```python
from build123d import *

# Parameters (mm, degrees)
FILLET1_R     = 1
CHAMFER1_SIZE = 0.5


with BuildPart() as part:
    # Sketch1 → Revolve1 (revolve)
    with BuildSketch(Plane.XY, mode=Mode.PRIVATE) as revolve1_sk:
        Polygon((-26, 0), (-22.5, 0), (-22.5, 2.872417267), (-15.5, 11.5), (-13, 11.5), (-13, 19.5), (-15.142082361, 19.5), (-25, 7.35), (-25, 1), (-26, 1), align=None)
    revolve(revolve1_sk.sketch.rotate(Axis((0, 0, 0), (0, 1, 0)), 270), axis=Axis((0, 0, 0), (0, 1, 0)))

    # Fillet1
    fillet1_edges = [part.edges().sort_by_distance(p)[0] for p in [
        (0, 2.872417267, 22.5),
        (0, 19.5, 15.142082361),
    ]]
    fillet(fillet1_edges, radius=FILLET1_R)

    # Chamfer1
    chamfer1_edges = [part.edges().sort_by_distance(p)[0] for p in [
        (0, 0, 22.5),
        (0, 0, 26),
    ]]
    chamfer(chamfer1_edges, length=CHAMFER1_SIZE)


solid = part.part
```
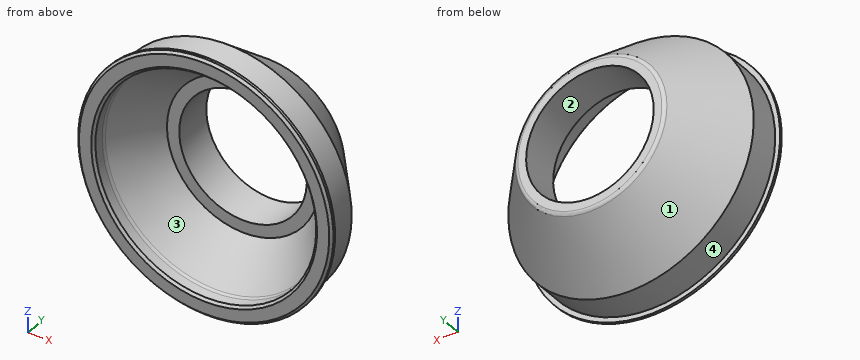
Can you work these out from the model? Positions are in its coordinate system, mm. Face numbers are marked on the shaded views. A direction names the side the tool comes from. Give positions to 0.01 mm unless a question says otherwise; leave off trailing zeros. Loops run counter-clockwise (first coordinate to the right, second up) from the corner with the lowest first, then second, coordinate; pieces in that order, holes last. Notation, with made-up numbers: M 51.25,-11.5 L 70.25,-11.5 A13 cw 70.25,-6.5 Z; hole C 79.25,19.5 d10. An arc over 180 degrees is marked long. One line per question, with ' | ' between items. Start each with the question number.
Q1. For the marked faces 3 and 4, which set-ups out of +Z, -Z, +X, -X, +Y, -Y let a thin tool reach every point of the face, with its end or its side?
Q2. If we section it at B-B (y = 9): Please give me the cut outline in (x, z), plus the area to 3 significant figures.
Q3. If we mould it in two halves opening along X, with no side actions, what happens to the marked faces 1 and 2? For each: +X half, -X half, draft (parallel to the pull), parting line (faces both ways), or undercut.
Q4. For pin 1 Ø5 at (x, y) = (-6.5, 12) entering from +Z; pin 2 Ø9.5 at (x, z) = (3, -2) entering from -Y; pin 3 Ø6 at (y, z) = (16, 2.5) entering from -X; pin 4 Ø8 at (y, z) = (2.5, -17) entering from -X, each with a flat end and sliding along its axis, tell me the tip position at first contact or that it passes through.
Q5. If I drill on line 1 (X direction, y = 1.1, z = 0); line 2 (X direction, y = 18.25, z = 0); line 3 (Z direction, x = -5.5, y = 18.75), over which ranges is the centre line in solid material (lowest first)? Write a range as from..to.
Q6. If we section it at A-A (y = 15.25): Please give me the cut outline in (x, z), plus the area to 3 significant figures.
Computed:
1) face 3: -Y | face 4: +Y
2) outline: C 0,0 d47.32; hole C 0,0 d35.06 | area: 794 mm²
3) face 1: parting line | face 2: undercut
4) pin 1: stops at z = 22.44 | pin 2: passes through | pin 3: stops at x = -20.29 | pin 4: stops at x = -22.35
5) line 1: x = -25..-22.5, 22.5..25 | line 2: x = -16.16..-13, 13..16.16 | line 3: z = -14.76..-11.78, 11.78..14.76
6) outline: C 0,0 d37.18; hole C 0,0 d26 | area: 555 mm²
